The model under review builds one solid part; all positions refer to its coordinate system, in mm. Face numbers are marked on the shaded views. A direction names the side the tool comes from. Give positions to 0.01 mm unless a question says otherwise; leave off trailing zeros. Order: outer loops, then holes, each group sorted by start corner. A loop starts at its lowest first (then second) coordinate and runs counter-clockwise, first axis right, second up. Notation, with made-up numbers: (77.5, 77) - (135.5, 77) arc R31 ccw to (135.5, 107) - close; hole circle Ø11 at (63.25, -31.5). An arc over 180 degrees is marked (long way). Use CSV: the item, a comma, the result in double quotes. Start each with the question number.
1. Draft analysis for pull direction Z (two halves, no side actions). For the marked faces 4, 5 and 6, state which applies: released by +Z, released by -Z, zero draft, split by the parting line, or undercut.
2. Take a section at B-B, the plane y = 6.25. State the section outline as (x, z) points, then the cut area to 3 significant figures.
3. Machinability: for the marked faces 1, 2 and 3, which of the approach directions +Z, -Z, +X, -X, +Y, -Y give a long, thin tool a straight path to every point of the face, cutting with its end or side? Answer none if there is none.
4. Take a section at A-A, the plane y = 8. State the section outline as (x, z) points, then the cut area to 3 significant figures.
5. To check wall thickness, follow line 1 (Y direction, x = 5.5, z = -7.5); line 2 (Y direction, x = 3.5, z = -1.25); line 3 (Z direction, x = -2.75, y = 4). State the ranges of each line that lie inside material, in increasing order. Write a range as [from, to].
6. For pin 1 (6 mm diameter, centred on x = 0, z = 9.5, fed in from +Y); pin 2 (3 mm diameter, centred on x = 2, z = -10.5, fed in from +Y); pin 3 (0.8 mm diameter, centred on x = 0, z = 4, fed in from -Y); pin 4 (2 mm diameter, centred on y = 6.5, z = -8, fed in from +X), all flat-tipped, find the tip position at first contact; note any pin that passes through.
```python
from build123d import *

# Parameters (mm, degrees)
BOSS_EXTRUDE1_DEPTH      = 1
BOSS_EXTRUDE2_DEPTH      = 0.6
BOSS_EXTRUDE2_TAPER      = 20
SKETCH4_W                = 9
SKETCH4_H                = 9.6
BOSS_EXTRUDE3_DEPTH      = 4
BOSS_EXTRUDE3_TAPER      = 10
CUT_EXTRUDE1_DEPTH       = 2
BOSS_EXTRUDE4_DEPTH      = 4
BOSS_EXTRUDE4_DEPTH_BACK = 4
BOSS_EXTRUDE5_DEPTH      = 4.218382
BOSS_EXTRUDE5_DEPTH_BACK = 4.218382
CUT_EXTRUDE2_DEPTH       = 3
CUT_EXTRUDE2_DEPTH_BACK  = 3


with BuildPart() as part:
    # Sketch1 → Boss-Extrude1 (new body)
    with BuildSketch(Plane(origin=(0, 0, 0), x_dir=(1, 0, 0), z_dir=(0, 1, 0))):
        with BuildLine():
            Line((8, 10.3), (8, 12.5))
            ThreePointArc((8, 12.5), (7.560660172, 13.560660172), (6.5, 14))
            Line((6.5, 14), (-6.5, 14))
            ThreePointArc((-6.5, 14), (-7.560660172, 13.560660172), (-8, 12.5))
            Line((-8, 12.5), (-8, -12.5))
            ThreePointArc((-8, -12.5), (-7.560660172, -13.560660172), (-6.5, -14))
            Line((-6.5, -14), (6.5, -14))
            ThreePointArc((6.5, -14), (7.560660172, -13.560660172), (8, -12.5))
            Line((8, -12.5), (8, 0.7))
            ThreePointArc((8, 0.7), (7.912132034, 0.912132034), (7.7, 1))
            Line((7.7, 1), (7.5, 1))
            ThreePointArc((7.5, 1), (7.287867966, 1.087867966), (7.2, 1.3))
            Line((7.2, 1.3), (7.2, 9.7))
            ThreePointArc((7.2, 9.7), (7.287867966, 9.912132034), (7.5, 10))
            Line((7.5, 10), (7.7, 10))
            ThreePointArc((7.7, 10), (7.912132034, 10.087867966), (8, 10.3))
        make_face()
    extrude(amount=BOSS_EXTRUDE1_DEPTH)

    # Sketch2 → Boss-Extrude2 (add)
    with BuildSketch(Plane(origin=(0, 1, 0), x_dir=(1, 0, 0), z_dir=(0, 1, 0))):
        Polygon((-8, 4.6), (-5, 4.6), (-5, -14), (-4, -14), (-4, 4.6), (-4, 6.4), (-4, 14), (-5, 14), (-5, 6.4), (-8, 6.4), align=None)
        Polygon((7.2, 4.6), (7.2, 6.4), (5, 6.4), (5, 14), (4, 14), (4, 6.4), (4, 4.6), (4, -14), (5, -14), (5, 4.6), align=None)
    extrude(amount=BOSS_EXTRUDE2_DEPTH, taper=BOSS_EXTRUDE2_TAPER)

    # Sketch4 → Boss-Extrude3 (add)
    with BuildSketch(Plane(origin=(0, 1, 0), x_dir=(1, 0, 0), z_dir=(0, 1, 0))):
        with Locations((0, -1.6)):
            Rectangle(SKETCH4_W, SKETCH4_H)
    extrude(amount=BOSS_EXTRUDE3_DEPTH, taper=BOSS_EXTRUDE3_TAPER)

    # Sketch5 → Cut-Extrude1 (cut)
    with BuildSketch(Plane(origin=(0, 5, 0), x_dir=(1, 0, 0), z_dir=(0, 1, 0))):
        with BuildLine():
            Line((-2.994692077, 1.994692077), (-1.025106513, 1.994692077))
            ThreePointArc((-1.025106513, 1.994692077), (0, -2.994692077), (1.025106513, 1.994692077))
            Line((1.025106513, 1.994692077), (2.994692077, 1.994692077))
            Line((2.994692077, 1.994692077), (2.994692077, 2.494692077))
            Line((2.994692077, 2.494692077), (2.994692077, 3.2))
            Line((2.994692077, 3.2), (-2.994692077, 3.2))
            Line((-2.994692077, 3.2), (-2.994692077, 2.494692077))
            Line((-2.994692077, 2.494692077), (-2.994692077, 1.994692077))
        make_face()
    extrude(amount=-CUT_EXTRUDE1_DEPTH, mode=Mode.SUBTRACT)

    # Sketch6 → Boss-Extrude4 (add, two sides)
    with BuildSketch(Plane(origin=(0, 0, 0), x_dir=(0, 0, -1), z_dir=(1, 0, 0))) as boss_extrude4_sk:
        with BuildLine():
            Line((-0.5, 0), (10.297970476, 9.67749108))
            ThreePointArc((10.297970476, 9.67749108), (13.042905373, 5.180705941), (14, 0))
            Line((14, 0), (-0.5, 0))
        make_face()
    extrude(amount=BOSS_EXTRUDE4_DEPTH)
    extrude(boss_extrude4_sk.sketch, amount=-BOSS_EXTRUDE4_DEPTH_BACK)

    # Sketch7 → Boss-Extrude5 (add, two sides)
    with BuildSketch(Plane(origin=(0, 0, 0), x_dir=(0, 0, -1), z_dir=(1, 0, 0))) as boss_extrude5_sk:
        with BuildLine():
            Line((2.970774925, 2.3), (7.731260017, 2.3))
            ThreePointArc((7.731260017, 2.3), (7.836854365, 2.323409703), (7.922661977, 2.3892522))
            Line((7.922661977, 2.3892522), (9.61889819, 4.4107478))
            ThreePointArc((9.61889819, 4.4107478), (9.704705802, 4.476590297), (9.81030015, 4.5))
            Line((9.81030015, 4.5), (13.464837448, 4.5))
            ThreePointArc((13.464837448, 4.5), (13.633638738, 4.434356768), (13.713744179, 4.271919003))
            Line((13.713744179, 4.271919003), (14, 1))
            Line((14, 1), (3.2, 1))
            Line((3.2, 1), (2.970774925, 2.3))
        make_face()
    extrude(amount=BOSS_EXTRUDE5_DEPTH)
    extrude(boss_extrude5_sk.sketch, amount=-BOSS_EXTRUDE5_DEPTH_BACK)

    # Sketch9 → Cut-Extrude2 (cut, two sides)
    with BuildSketch(Plane(origin=(0, 0, 0), x_dir=(0, 0, -1), z_dir=(1, 0, 0))) as cut_extrude2_sk:
        with BuildLine():
            ThreePointArc((9.226818428, 4.426818428), (9.30787804, 4.480980729), (9.403494371, 4.5))
            Line((9.403494371, 4.5), (11.8219778, 4.5))
            ThreePointArc((11.8219778, 4.5), (11.97560279, 4.447191058), (12.064288583, 4.311087229))
            ThreePointArc((12.064288583, 4.311087229), (12.315752859, 2.965896786), (12.4, 1.6))
            Line((12.4, 1.6), (12.4, 0))
            Line((12.4, 0), (-5.6, 0))
            Line((-5.6, 0), (-5.6, 1.5781403))
            ThreePointArc((-5.6, 1.5781403), (-5.599049217, 1.599916817), (-5.596204103, 1.621527602))
            Line((-5.596204103, 1.621527602), (-5.495344685, 2.193529787))
            ThreePointArc((-5.495344685, 2.193529787), (-5.409888382, 2.341544446), (-5.249283067, 2.4))
            Line((-5.249283067, 2.4), (-2.562432787, 2.4))
            ThreePointArc((-2.562432787, 2.4), (-2.466816455, 2.380980729), (-2.385756844, 2.326818428))
            Line((-2.385756844, 2.326818428), (-1.732119987, 1.673181572))
            ThreePointArc((-1.732119987, 1.673181572), (-1.651060376, 1.619019271), (-1.555444044, 1.6))
            Line((-1.555444044, 1.6), (6.296505629, 1.6))
            ThreePointArc((6.296505629, 1.6), (6.39212196, 1.619019271), (6.473181572, 1.673181572))
            Line((6.473181572, 1.673181572), (9.226818428, 4.426818428))
        make_face()
    extrude(amount=CUT_EXTRUDE2_DEPTH, mode=Mode.SUBTRACT)
    extrude(cut_extrude2_sk.sketch, amount=-CUT_EXTRUDE2_DEPTH_BACK, mode=Mode.SUBTRACT)


solid = part.part
```
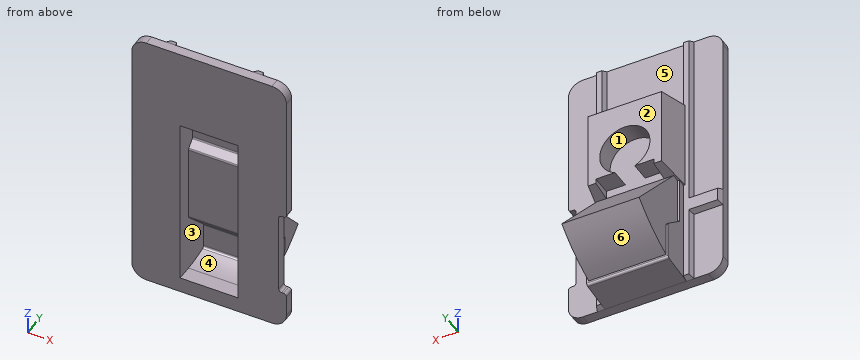
Determined:
1,face 4,"undercut"
1,face 5,"zero draft"
1,face 6,"released by -Z"
2,outline,"(-4, -12.58) - (4, -12.58) - (4, -6.47) - (-4, -6.47) - close"
2,area,"48.9 mm²"
3,face 1,"+Y"
3,face 2,"+Z, +X, -X, +Y"
3,face 3,"-Y"
4,outline,"(-4, -11.59) - (4, -11.59) - (4, -8.43) - (-4, -8.43) - close"
4,area,"25.3 mm²"
5,line 1,"y = [0, 1]"
5,line 2,"y = [0, 5]"
5,line 3,"z = [-13.74, -12.14], [-8.8, -3.96], [-1.99, 5.87]"
6,pin 1,"stops at y = 1"
6,pin 2,"stops at y = 9.68"
6,pin 3,"stops at y = 2.4"
6,pin 4,"stops at x = 4"
